Work out the finished part from the listing and answer in its coordinate system (mm). Face numbers are marked on the shaded views. A direction names the side the tool comes from. Coordinates: 2 decimals unless noted, no trailing zeros. Order: outer loops, then holes, each group sorted by start corner. A loop starts at its lowest first (then second) coordinate and runs counter-clockwise, first axis right, second up.
1. The part is cut by section A-A, the plane x = -220. Give the vertices of the cut face in (y, z), then the cut area to 3 significant figures.
2. Find the intervals of material crossed by probe 1 along X at (y, z) = (257, -66); probe 2 along Y at (x, z) = (1.5, 196.5); probe 3 along Z at (x, y) = (187, 295), in increasing order.
3. The part is cut by section B-B, the plane z = -190.5. Give the vertices of the cut face in (x, y).
4. Flat-ended cylindrical pins translate along their axes: pin 1 Ø8 at (x, y) = (80, 286) entering from -Z; pin 2 Ø4 at (x, z) = (-47, 109) entering from -Y. Find the tip coordinate at first contact, or state that the pin passes through.
5. A tool of negligible diameter and unlimited length cuts with its end or side. For the marked faces 1 and 2, from which of +Z, -Z, +X, -X, +Y, -Y can it reach the whole face along a straight path? Write none if from no direction.
6. The part is cut by section C-C, the plane y = 39. Give the vertices of the cut face in (x, z), then the cut area to 3 significant figures.
7. Determine the mould class of the marked faces 3, 4 and 5 for opening direction X: +X half, -X half, draft (parallel to the pull), parting line (faces both ways), or undercut.
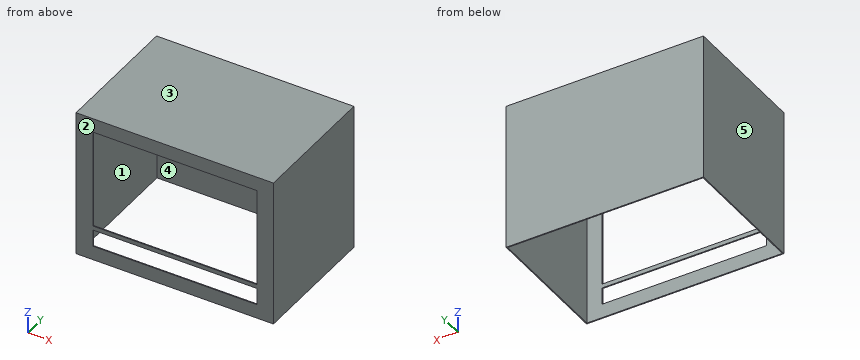
```python
from build123d import *

# Parameters (mm, degrees)
F0_W     = 600
F0_H     = 450
F0_W_2   = 500
F0_H_2   = 51.817134
F0_H_3   = 300
F1_DEPTH = 400
F2_T     = -3
F3_DEPTH = 3


with BuildPart() as f1:
    # F0 (on Front) → F1 (new body)
    with BuildSketch(Plane.XZ):
        Rectangle(F0_W, F0_H)
        with Locations((0.704244, -156.171255)):
            Rectangle(F0_W_2, F0_H_2, mode=Mode.SUBTRACT)
        with Locations((0.704244, 32.232778)):
            Rectangle(F0_W_2, F0_H_3, mode=Mode.SUBTRACT)
        with Locations((0.704244, 32.232778)):
            Rectangle(F0_W_2, F0_H_3)
        with Locations((0.704244, -156.171255)):
            Rectangle(F0_W_2, F0_H_2)
    extrude(amount=-F1_DEPTH)

    # F2
    f2_openings = [f1.faces().sort_by_distance(p)[0] for p in [
        (0, 200, -225),
    ]]
    offset(amount=F2_T, openings=f2_openings)

    # F0 (on Front) → F3 (cut)
    with BuildSketch(Plane.XZ):
        with Locations((0.704244, 32.232778)):
            Rectangle(F0_W_2, F0_H_3)
        with Locations((0.704244, -156.171255)):
            Rectangle(F0_W_2, F0_H_2)
    extrude(amount=-F3_DEPTH, mode=Mode.SUBTRACT)


solid = f1.part
```
Geometry says:
1. outline: (0, -225) - (3, -225) - (3, -182.08) - (0, -182.08) - close; (0, -130.26) - (3, -130.26) - (3, -117.77) - (0, -117.77) - close; (0, 182.23) - (3, 182.23) - (3, 222) - (397, 222) - (397, -225) - (400, -225) - (400, 225) - (0, 225) - close
1. area: 2,830 mm2
2. probe 1: x = -300 to -297, 297 to 300
2. probe 2: y = 0 to 3, 397 to 400
2. probe 3: z = 222 to 225
3. outline: (-300, 0) - (300, 0) - (300, 400) - (-300, 400) - close; hole (-297, 3) - (297, 3) - (297, 397) - (-297, 397) - close
4. pin 1: stops at z = 222
4. pin 2: stops at y = 397
5. face 1: -Z
5. face 2: +Z, -Z, +X, -X, -Y
6. outline: (-300, -225) - (-297, -225) - (-297, 222) - (297, 222) - (297, -225) - (300, -225) - (300, 225) - (-300, 225) - close
6. area: 4,480 mm2
7. face 3: draft
7. face 4: undercut
7. face 5: -X half
